```python
from build123d import *

# Parameters (mm, degrees)
F1_DEPTH = 23
F2_R     = 0.5
F3_DEPTH = 6


with BuildPart() as f1:
    # F0 (on Front) → F1 (new body)
    with BuildSketch(Plane.XZ):
        Polygon((0, 14), (-41.842094, 14), (-41.842094, 0), (0, 0), (0, 5), (-39.091877, 5), (-39.302094, 8.994472), (0, 8.994472), align=None)
    extrude(amount=F1_DEPTH)

    # F2 (on Right) → F3 (cut)
    with BuildSketch(Plane.YZ):
        with Locations((-12, 10.408686)):
            Circle(F2_R)
        with Locations((-12, 3.5)):
            Circle(F2_R)
    extrude(amount=-F3_DEPTH, mode=Mode.SUBTRACT)


solid = f1.part
```
Geometry: final body of the model. Coordinates: model frame, mm. A direction names the side the tool comes from. Give positions to 0.01 mm unless a question says otherwise; leave off trailing zeros. Loops run counter-clockwise (first coordinate to the right, second up) from the corner with the lowest first, then second, coordinate; pieces in that order, holes last. Notation, with made-up numbers: (-26, 12.25) -> (10, 12.25) arc R12 cw to (10, 20.25) -> close; hole circle Ø11 at (41, 75). An arc over 180 degrees is marked (long way). Use one line per item in the form item = value.
Item 1: Section query D-D on y = -9.5. Output: boundary loops of the cut face in (x, z), and give its area (3 significant figures).
A:
outline = (-41.84, 0) -> (0, 0) -> (0, 5) -> (-39.09, 5) -> (-39.3, 8.99) -> (0, 8.99) -> (0, 14) -> (-41.84, 14) -> close
area = 429 mm^2
Item 2: Section query C-C on x = -5.5. Output: boundary loops of the cut face in (y, z).
A:
outline = (-23, 0) -> (0, 0) -> (0, 5) -> (-23, 5) -> close; (-23, 8.99) -> (0, 8.99) -> (0, 14) -> (-23, 14) -> close; hole circle Ø1 at (-12, 3.5); hole circle Ø1 at (-12, 10.41)
Item 3: Section query A-A on x = -25. Output: boundary loops of the cut face in (y, z), and give its area (3 significant figures).
A:
outline = (-23, 0) -> (0, 0) -> (0, 5) -> (-23, 5) -> close; (-23, 8.99) -> (0, 8.99) -> (0, 14) -> (-23, 14) -> close
area = 230 mm^2
Item 4: Access query for faces 5 (the face through (-39.196, -11.339, 6.969)), 6 (the face through (-41.842, -11, 7)), 7 (the face through (-6, -12, 10.4)). Directions: +Z, -Z, +X, -X, +Y, -Y. A direction counts if a zero-diameter tool reaches every point of the face in a straight line with its end or side. Return the directions, or none.
A:
face_5 = +X, +Y, -Y
face_6 = +Z, -Z, -X, +Y, -Y
face_7 = +X
Item 5: Section query B-B on y = -12. Output: boundary loops of the cut face in (x, z).
A:
outline = (-41.84, 0) -> (0, 0) -> (0, 3) -> (-6, 3) -> (-6, 4) -> (0, 4) -> (0, 5) -> (-39.09, 5) -> (-39.3, 8.99) -> (0, 8.99) -> (0, 9.91) -> (-6, 9.91) -> (-6, 10.91) -> (0, 10.91) -> (0, 14) -> (-41.84, 14) -> close
Item 6: Pin query (flat end, axial travel): P1, Ø1, axis at x = -17.5, z = 9, coming from the +Y side; P2, Ø0.5, axis at y = -12, z = 10.5, coming from the +X side. Return the tip coordinate at first contact, or that it passes through.
A:
P1 = 0
P2 = -6
Item 7: Draft query along Y for faces 1 (the face through (-6, -12, 3.5)), 2 (the face through (-3, -12.1, 10.9)), 3 (the face through (-21, 0, 4)), 4 (the face through (0, -11, 11)). Return one class per face: pulls with the +Y half, pulls with the -Y half, needs draft (parallel to the pull), parting line crosses it, or undercut.
A:
face_1 = undercut
face_2 = undercut
face_3 = pulls with the +Y half
face_4 = needs draft
Item 8: Line query: probe 1 along Z at (x, y) = (-1.3, -12); probe 2 along Z at (x, y) = (-19, -2.5); probe 3 along Y at (x, z) = (-2, 10). Output: solid intervals per line, ascending.
A:
probe_1 = 0 to 3, 4 to 5, 8.99 to 9.91, 10.91 to 14
probe_2 = 0 to 5, 8.99 to 14
probe_3 = -23 to -12.29, -11.71 to 0
